Read the model definition and answer for the solid it produces. Units are mm, in the model's axes. A direction names the side the tool comes from. Give positions to 0.01 mm unless a question says otherwise; leave off trailing zeros. Write each loop counter-clockwise with the first axis right and the second up, starting at its lowest first coordinate (ties: lowest second). Pieces come first, ordered by that corner, then holes. Notation, with made-up numbers: (55.5, -4) - (65.5, -4) arc R11 ccw to (65.5, 16) - close; hole circle Ø6 at (22, 71.25). An arc over 180 degrees is marked (long way). Answer as a JSON object with one key per item and string values. Group by question number.
```python
from build123d import *

# Parameters (mm, degrees)
SKETCH_2_OUTSIDE_W  = 21.352
SKETCH_2_OUTSIDE_H  = 21.352
CUT_EXTRUDE_1_DEPTH = 19
HOLE_WIZARD_M4_1_D  = 3.3
SKETCH_5_R          = 3
CUT_EXTRUDE_2_DEPTH = 14
HOLE_WIZARD_M3_1_D  = 2.5


with BuildPart() as part:
    # 草图1 → 旋转1 (revolve)
    with BuildSketch(Plane.XY):
        Polygon((0, 0), (0, 18), (7, 18), (7, 12), (5.5, 12), (5.5, 0), align=None)
    revolve(axis=Axis((0, 0, 0), (0, 1, 0)))

    # 草图2 outside → 切除-拉伸1 (cut, through all)
    with BuildSketch(Plane(origin=(0, 18, 0), x_dir=(1, 0, 0), z_dir=(0, 1, 0))):
        Rectangle(SKETCH_2_OUTSIDE_W, SKETCH_2_OUTSIDE_H)
        Polygon((7.101408311, 0), (3.550704156, 6.15), (-3.550704156, 6.15), (-7.101408311, 0), (-3.550704156, -6.15), (3.550704156, -6.15), align=None, mode=Mode.SUBTRACT)
    extrude(amount=-CUT_EXTRUDE_1_DEPTH, mode=Mode.SUBTRACT)

    # M4 螺纹孔1 (through all)
    with Locations(Plane(origin=(0, 18, 0), x_dir=(1, 0, 0), z_dir=(0, 1, 0))):
        with Locations((0, 0)):
            Hole(HOLE_WIZARD_M4_1_D / 2)

    # 草图5 → 切除-拉伸2 (cut)
    with BuildSketch(Plane.XZ):
        Circle(SKETCH_5_R)
    extrude(amount=-CUT_EXTRUDE_2_DEPTH, mode=Mode.SUBTRACT)

    # M3 螺纹孔1 (through all)
    with Locations(Plane(origin=(-2.75, 0, 4.763139721), x_dir=(-0.866025404, 0, -0.5), z_dir=(-0.5, 0, 0.866025404))):
        with Locations((0, -4)):
            Hole(HOLE_WIZARD_M3_1_D / 2)


solid = part.part
```
1) Find the intervals of material crossed by line 1 (Z direction, x = 0, y = 16.5); line 2 (Z direction, x = 0, y = 10.25); line 3 (Y direction, x = -5.75, z = 0), in increasing order. Write a range as [from, to].
2) Flat-ended cylindrical pins translate along their axes: pin 1 Ø3 at (x, y) = (-4.5, 5) entering from +Z; pin 2 Ø3 at (y, z) = (16, 3) entering from +X. Find the tip coordinate at first contact, or state that the pin passes through.
3) For a pull along Z with two mould halves and no side action, classify faces 3 (the cylindrical face through (1.384, 6.902, -2.662)), 4 (the flat face through (-4, 12, -4)), 5 (the flat face through (5.3, 15.04, 3.12)) as released by +Z, released by -Z, zero draft, split by the parting line, or undercut.
4) Find section D-D, the plane x = 4.25. Write down the section's boundary in (y, z).
5) Find section A-A, the plane x = 0. Write down the section's boundary in (y, z).
6) Find section B-B, the plane y = 14.5. Write down the section's boundary in (x, z).
7) Which of the six approach directions +Z, -Z, +X, -X, +Y, -Y give full straight-line access (tool end or side, diameter ignored) to faces 1 (the cylindrical face through (-1.19, 5.92, 5.37)), 2 (the cylindrical face through (1.21, 4.76, -4.08))?
8) Find section C-C, the plane z = 0.5. Write down the section's boundary in (x, y).
Values follow:
{
 "1": {"line 1": "z = [-6.15, -1.65], [1.65, 6.15]", "line 2": "z = [-5.5, -3], [3, 5.5]", "line 3": "y = [12, 18]"},
 "2": {"pin 1": "stops at z = 4.6", "pin 2": "stops at x = 6.24"},
 "3": {"face 3": "undercut", "face 4": "zero draft", "face 5": "released by +Z"},
 "4": {"outline": "(0, -3.49) - (12, -3.49) - (12, -4.94) - (18, -4.94) - (18, 4.94) - (12, 4.94) - (12, 3.49) - (0, 3.49) - close"},
 "5": {"outline": "(0, -5.5) - (12, -5.5) - (12, -6.15) - (18, -6.15) - (18, -1.65) - (14, -1.65) - (14, -3) - (0, -3) - close; (0, 3) - (14, 3) - (14, 1.65) - (18, 1.65) - (18, 6.15) - (12, 6.15) - (12, 5.5) - (0, 5.5) - close"},
 "6": {"outline": "(-7, -0.18) - (-3.65, -5.97) arc R7 ccw to (-3.34, -6.15) - (3.34, -6.15) arc R7 ccw to (3.65, -5.97) - (7, -0.18) arc R7 ccw to (7, 0.18) - (3.65, 5.97) arc R7 ccw to (3.34, 6.15) - (-3.34, 6.15) arc R7 ccw to (-3.65, 5.97) - (-7, 0.18) arc R7 ccw to start; hole circle Ø3.3 at (0, 0)"},
 "7": {"face 1": "-Y", "face 2": "none"},
 "8": {"outline": "(-6.81, 12) - (-5.48, 12) - (-5.48, 0) - (-2.96, 0) - (-2.96, 14) - (-1.57, 14) - (-1.57, 18) - (-6.81, 18) - close; (1.57, 14) - (2.96, 14) - (2.96, 0) - (5.48, 0) - (5.48, 12) - (6.81, 12) - (6.81, 18) - (1.57, 18) - close"}
}
